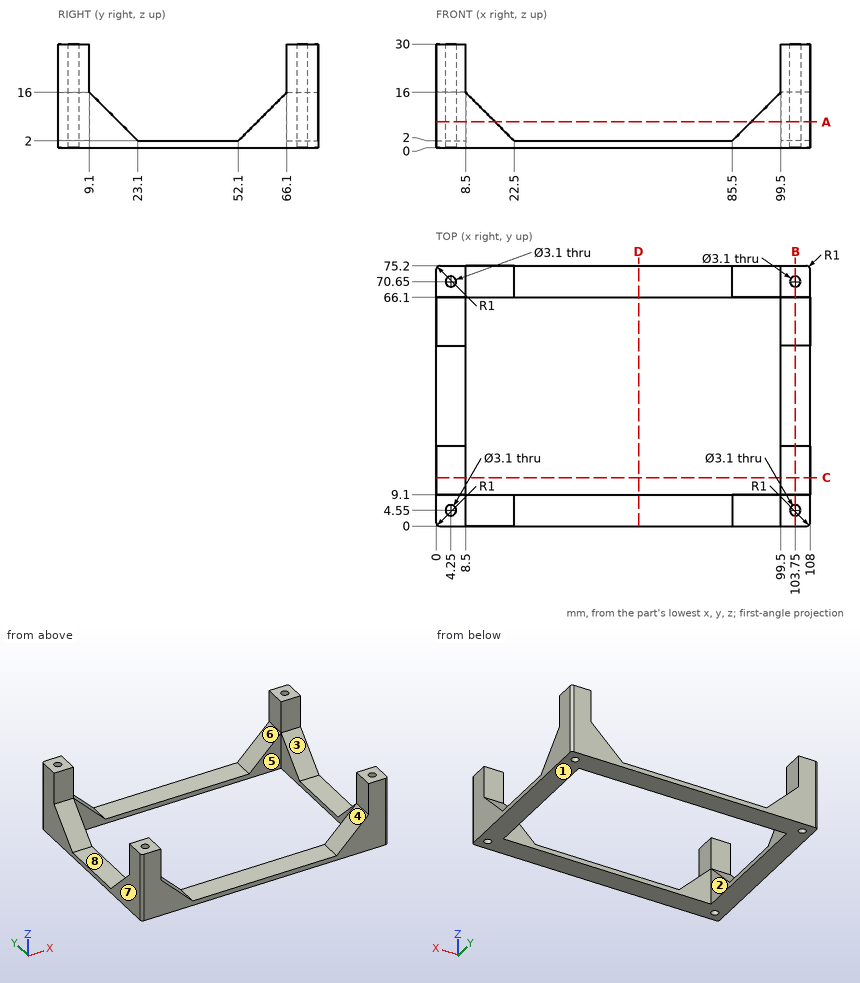
Answer from the drawing. Dimensions are ordinates in mm from the lowest x, y and z of the part. A direction names the side the tool comes from. Give positions to 0.01 mm unless a question says otherwise; leave off trailing zeros. Loops run counter-clockwise (first coordinate to the right, second up) from the corner with the lowest first, then second, coordinate; pieces in that order, holes last. Notation, with made-up numbers: (-26.5, 29) -> (12.5, 29) arc R25 cw to (12.5, 59) -> close; hole circle Ø4 at (15.5, 73.5). An arc over 180 degrees is marked (long way). Use a Markdown table: item, result.
Q1. Section D-D, the plane x = 58.5 is taken. Determine the outline of the cut face in (y, z), then the cut area to 3 significant figures.
Solved:
| item | result |
|---|---|
| outline | (0, 0) -> (9.1, 0) -> (9.1, 2) -> (0, 2) -> close; (66.1, 0) -> (75.2, 0) -> (75.2, 2) -> (66.1, 2) -> close |
| area | 36.4 mm^2 |
Q2. Determine the mould class of the marked faces 5, 6, 7 and 8 for opening direction X: pulls with the +X half, pulls with the -X half, needs draft (parallel to the pull), parting line crosses it, or undercut.
Solved:
| item | result |
|---|---|
| face 5 | undercut |
| face 6 | undercut |
| face 7 | pulls with the -X half |
| face 8 | needs draft |
Q3. A tool of negligible diameter and unlimited length cuts with its end or side. For the marked faces 1, 2, 3 and 4, from which of +Z, -Z, +X, -X, +Y, -Y can it reach the whole face along a straight path? Write none if from no direction.
Solved:
| item | result |
|---|---|
| face 1 | -Z, +X, -X, +Y, -Y |
| face 2 | +Z, -Z |
| face 3 | +Z, +X, -X |
| face 4 | +Z, +Y, -Y |
Q4. Section C-C, the plane y = 14 is taken. Determine the outline of the cut face in (x, z).
Solved:
| item | result |
|---|---|
| outline | (0, 0) -> (8.5, 0) -> (8.5, 11.1) -> (0, 11.1) -> close; (99.5, 0) -> (108, 0) -> (108, 11.1) -> (99.5, 11.1) -> close |
Q5. Section B-B, the plane x = 103.75 is taken. Determine the outline of the cut face in (y, z), then the cut area to 3 significant figures.
Solved:
| item | result |
|---|---|
| outline | (0, 0) -> (3, 0) -> (3, 30) -> (0, 30) -> close; (6.1, 0) -> (69.1, 0) -> (69.1, 30) -> (66.1, 30) -> (66.1, 16) -> (52.1, 2) -> (23.1, 2) -> (9.1, 16) -> (9.1, 30) -> (6.1, 30) -> close; (72.2, 0) -> (75.2, 0) -> (75.2, 30) -> (72.2, 30) -> close |
| area | 670 mm^2 |
Q6. Section A-A, the plane z = 7.5 is taken. Count the separate pieces of the cut face and the enclosed holes in it, then the cut area to 3 significant figures.
Solved:
| item | result |
|---|---|
| separate pieces | 4 |
| enclosed holes | 4 |
| area | 877 mm^2 |
Q7. This flat-tipped pin is pushed along its axis until it touches: pin 1 (7 mm diameter, centred on x = 104.5, y = 41.5, fed in from +Z). Where does it stop, or does it pass through?
Solved:
| item | result |
|---|---|
| pin 1 | stops at z = 2 |
Q8. Find the intervals of material crossed by line 1 along Y through (x, z) = (4.25, 20.5); line 2 along X through (y, z) = (70.65, 19.25); line 3 along X through (y, z) = (70.65, 15.25), in increasing order.
Solved:
| item | result |
|---|---|
| line 1 | y = 0 to 3, 6.1 to 9.1, 66.1 to 69.1, 72.2 to 75.2 |
| line 2 | x = 0 to 2.7, 5.8 to 8.5, 99.5 to 102.2, 105.3 to 108 |
| line 3 | x = 0 to 2.7, 5.8 to 9.25, 98.75 to 102.2, 105.3 to 108 |
